Source: CAD feature listing. Evaluate the final solid. Frame: model axes, mm. A direction names the side the tool comes from. Give positions to 0.01 mm unless a question says otherwise; leave off trailing zeros. Order: outer loops, then holes, each group sorted by start corner. A loop starts at its lowest first (then second) coordinate and runs counter-clockwise, first axis right, second up.
from build123d import *

# Parameters (mm, degrees)
CONG_1_R                = 1
ESQUISSE2_W             = 17
ESQUISSE2_H             = 10
BOSS_EXTRU_1_DEPTH      = 20
CONG_2_R                = 1
ENL_V_MAT_EXTRU_1_REACH = 40.962
ESQUISSE5_R             = 3
BOSS_EXTRU_2_DEPTH      = 7
CHANFREIN1_SIZE         = 1
CHANFREIN2_SIZE         = 1


with BuildPart() as part:
    # Esquisse1 → Révolution1 (revolve)
    with BuildSketch(Plane.XY, mode=Mode.PRIVATE) as r_volution1_sk:
        Polygon((-12, 0), (-12, 9), (0, 9), (0, 11), (-14, 11), (-14, 0), align=None)
    revolve(r_volution1_sk.sketch.rotate(Axis((0, 0, 0), (0, 1, 0)), 270), axis=Axis((0, 0, 0), (0, 1, 0)))

    # Congé1
    cong_1_edges = [part.edges().sort_by_distance(p)[0] for p in [
        (0, 11, 14),
    ]]
    fillet(cong_1_edges, radius=CONG_1_R)

    # Esquisse2 → Boss.-Extru.1 (add)
    with BuildSketch(Plane(origin=(0, 11, 0), x_dir=(1, 0, 0), z_dir=(0, 1, 0))):
        Rectangle(ESQUISSE2_W, ESQUISSE2_H)
    extrude(amount=BOSS_EXTRU_1_DEPTH)

    # Congé2
    cong_2_edges = [part.edges().sort_by_distance(p)[0] for p in [
        (8.5, 11, 0),
        (0, 11, -5),
        (-8.5, 11, 0),
        (0, 11, 5),
    ]]
    fillet(cong_2_edges, radius=CONG_2_R)

    # Esquisse3 → Enlèv. mat.-Extru.1 (cut, up to next)
    with BuildSketch(Plane.XY.offset(5), mode=Mode.PRIVATE) as enl_v_mat_extru_1_sk1:
        with BuildLine():
            ThreePointArc((-8.5, 22.5), (-6.010407626, 28.510407654), (4e-08, 31))
            Line((4e-08, 31), (-8.5, 31))
            Line((-8.5, 31), (-8.5, 22.5))
        make_face()
    enl_v_mat_extru_1_tool1 = extrude(enl_v_mat_extru_1_sk1.sketch, amount=-ENL_V_MAT_EXTRU_1_REACH, mode=Mode.PRIVATE) & part.part
    # Esquisse3 → Enlèv. mat.-Extru.1 (cut, up to next)
    with BuildSketch(Plane.XY.offset(5), mode=Mode.PRIVATE) as enl_v_mat_extru_1_sk2:
        with BuildLine():
            ThreePointArc((4e-08, 31), (6.010407654, 28.510407626), (8.5, 22.5))
            Line((8.5, 22.5), (8.5, 31))
            Line((8.5, 31), (4e-08, 31))
        make_face()
    enl_v_mat_extru_1_tool2 = extrude(enl_v_mat_extru_1_sk2.sketch, amount=-ENL_V_MAT_EXTRU_1_REACH, mode=Mode.PRIVATE) & part.part
    add(enl_v_mat_extru_1_tool1.solids().sort_by_distance((-6.601373, 29.101373, 5))[0], mode=Mode.SUBTRACT)
    add(enl_v_mat_extru_1_tool2.solids().sort_by_distance((6.601373, 29.101373, 5))[0], mode=Mode.SUBTRACT)

    # Esquisse5 → Boss.-Extru.2 (add)
    with BuildSketch(Plane.XY.offset(5)):
        with Locations(Location((0, 26, 0), (0, 0, 180))):
            Circle(ESQUISSE5_R)
    boss_extru_2 = extrude(amount=BOSS_EXTRU_2_DEPTH)

    # Chanfrein1
    chanfrein1_edges = [part.edges().sort_by_distance(p)[0] for p in [
        (3, 26, 12),
    ]]
    chamfer(chanfrein1_edges, length=CHANFREIN1_SIZE)

    # Symétrie4: Boss.-Extru.2 across plane
    add(boss_extru_2.mirror(Plane.XY))

    # Chanfrein2
    chanfrein2_edges = [part.edges().sort_by_distance(p)[0] for p in [
        (3, 26, -12),
    ]]
    chamfer(chanfrein2_edges, length=CHANFREIN2_SIZE)


solid = part.part
1) Reachability of faces 1 (the face through (0.65, 28.93, 7.96)), 2 (the face through (8.5, 17, 0)), 3 (the face through (0.65, 28.93, -7.96)), 4 (the face through (0, 26, 12)), 5 (the face through (-3.604, 4.563, -11.446)) from +Z, -Z, +X, -X, +Y, -Y: full face, straight path, thin tool, end or side. Return the list, or none.
Checks:
face 1: +Z
face 2: +Z, -Z, +X, +Y
face 3: -Z
face 4: +Z, +X, -X, +Y
face 5: -Y
2) Section query A-A on y = 26. Output: boundary loops of the cut face in (x, z), and give its area (3 significant figures).
Checks:
outline: (-7.75, -5) - (-3, -5) - (-3, -11) - (-2, -12) - (2, -12) - (3, -11) - (3, -5) - (7.75, -5) - (7.75, 5) - (3, 5) - (3, 11) - (2, 12) - (-2, 12) - (-3, 11) - (-3, 5) - (-7.75, 5) - close
area: 237 mm2
3) Pull-direction query (Z, two-part tool) for faces 6 (the face through (8.801, 11.285, -0.084)), 7 (the face through (0, 9, 0)), 8 (the face through (13.67, 4.93, 3.03)); classes: +Z half, -Z half, draft (parallel to the pull), parting line (faces both ways), or undercut.
Checks:
face 6: draft
face 7: undercut
face 8: parting line
4) First-contact query: pin 1 Ø8 at (y, z) = (27.5, 6) entering from -X; pin 2 Ø3 at (x, y) = (3, 17) entering from +Z; pin 3 Ø5 at (y, z) = (24.5, 8) entering from +X. Flat tips, straight axial feed; report the tip coordinate or a pass-through.
Checks:
pin 1: stops at x = -8.42
pin 2: stops at z = 5
pin 3: stops at x = 3
5) Section query C-C on y = 4. Output: boundary loops of the cut face in (x, z), and give its area (3 significant figures).
Checks:
outline: circle Ø28 at (0, 0); hole circle Ø24 at (0, 0)
area: 163 mm2
6) Ray query, L1, parallel to X at y = 2.5, z = 0; L2, parallel to Z at x = 0.75, y = 17.5; L3, parallel to X at y = 12, z = -2. Return the intervals inside material, ascending.
Checks:
L1: x = -14 to -12, 12 to 14
L2: z = -5 to 5
L3: x = -8.5 to 8.5
7) Section query B-B on z = 0. Output: boundary loops of the cut face in (x, y), and give its area (3 significant figures).
Checks:
outline: (-14, 0) - (-12, 0) - (-12, 9) - (12, 9) - (12, 0) - (14, 0) - (14, 10) arc R1 ccw to (13, 11) - (9.5, 11) arc R1 cw to (8.5, 12) - (8.5, 22.5) arc R8.5 ccw to (-8.5, 22.5) - (-8.5, 12) arc R1 cw to (-9.5, 11) - (-13, 11) arc R1 ccw to (-14, 10) - close
area: 401 mm2
